Work out the finished part from the listing and answer in its coordinate system (mm). A direction names the side the tool comes from. Round coordinates to 2 decimals unless told otherwise and drop trailing zeros. Loops run counter-clockwise (first coordinate to the right, second up) from the corner with the lowest first, then second, coordinate; pieces in that order, holes last. Notation, with made-up numbers: (22, 84) - (47, 84) arc R8 cw to (47, 89) - close; hole circle Ø4 at (42.25, 51.5). An arc over 180 degrees is marked (long way). Return JSON: item names as keys, results as strings.
from build123d import *

# Parameters (mm, degrees)
BOSS_EXTRUDE1_DEPTH = 30
SKETCH2_R           = 1.5
SKETCH2_R_2         = 7.5
CUT_EXTRUDE1_DEPTH  = 14
SKETCH3_R           = 1.5
CUT_EXTRUDE2_DEPTH  = 76
FILLET1_R           = 5


with BuildPart() as part:
    # Sketch1 → Boss-Extrude1 (new body)
    with BuildSketch(Plane(origin=(0, 0, 0), x_dir=(1, 0, 0), z_dir=(0, 1, 0))):
        Polygon((-11.5, 4), (-1.5, 4), (-1.5, 75), (1.5, 75), (1.5, 4), (11.5, 4), (11.5, 0), (-11.5, 0), align=None)
    extrude(amount=BOSS_EXTRUDE1_DEPTH)

    # Sketch2 → Cut-Extrude1 (cut, through all)
    with BuildSketch(Plane.ZY.offset(1.5)):
        with Locations((-67.5, 15)):
            Circle(SKETCH2_R)
        with Locations((-31.5, 15)):
            Circle(SKETCH2_R)
        with Locations((-49.5, 15)):
            Circle(SKETCH2_R_2)
    extrude(amount=-CUT_EXTRUDE1_DEPTH, mode=Mode.SUBTRACT)

    # Sketch3 → Cut-Extrude2 (cut, through all)
    with BuildSketch(Plane.XY):
        with Locations((-6.5, 26)):
            Circle(SKETCH3_R)
        with Locations((-6.5, 4)):
            Circle(SKETCH3_R)
        with Locations((6.5, 4)):
            Circle(SKETCH3_R)
        with Locations((6.5, 26)):
            Circle(SKETCH3_R)
    extrude(amount=-CUT_EXTRUDE2_DEPTH, mode=Mode.SUBTRACT)

    # Fillet1
    fillet1_edges = [part.edges().sort_by_distance(p)[0] for p in [
        (11.5, 0, -2),
        (-11.5, 0, -2),
        (11.5, 30, -2),
        (0, 30, -75),
        (-11.5, 30, -2),
        (0, 0, -75),
    ]]
    fillet(fillet1_edges, radius=FILLET1_R)


solid = part.part
1) Section A-A (z = -67.5) is taken. Give the vertices of the cut face in (x, y), and give its area (3 significant figures).
Verdict:
{"outline": "(-1.5, 0) - (1.5, 0) - (1.5, 13.5) - (-1.5, 13.5) - close; (-1.5, 16.5) - (1.5, 16.5) - (1.5, 30) - (-1.5, 30) - close", "area": "81.0 mm2"}
2) Section B-B (y = 15) is taken. Give the vertices of the cut face in (x, z).
Verdict:
{"outline": "(-11.5, -4) - (-1.5, -4) - (-1.5, -30) - (1.5, -30) - (1.5, -4) - (11.5, -4) - (11.5, 0) - (-11.5, 0) - close; (-1.5, -75) - (1.5, -75) - (1.5, -69) - (-1.5, -69) - close; (-1.5, -66) - (1.5, -66) - (1.5, -57) - (-1.5, -57) - close; (-1.5, -42) - (1.5, -42) - (1.5, -33) - (-1.5, -33) - close"}
3) Flat-ended cylindrical pins translate along their axes: pin 1 (8 mm diameter, centred on y = 23, z = -66.5, fed in from +X); pin 2 (5 mm diameter, centred on x = 6.5, y = 26, fed in from -Z); pin 3 (3 mm diameter, centred on y = 20, z = -39.5, fed in from -X). Find the tip coordinate at first contact, or state that the pin passes through.
Verdict:
{"pin 1": "stops at x = 1.5", "pin 2": "stops at z = -4", "pin 3": "stops at x = -1.5"}
4) Section D-D (y = 4) is taken. Give the vertices of the cut face in (x, z).
Verdict:
{"outline": "(-11.4, -4) - (-8, -4) - (-8, 0) - (-11.4, 0) - close; (-5, -4) - (-1.5, -4) - (-1.5, -74.9) - (1.5, -74.9) - (1.5, -4) - (5, -4) - (5, 0) - (-5, 0) - close; (8, -4) - (11.4, -4) - (11.4, 0) - (8, 0) - close"}
5) Find the intervals of material crossed by L1, parallel to Y at x = 0.5, z = -67.5; L2, parallel to Y at x = -0.7, z = -49.5; L3, parallel to Z at x = 4.5, y = 6, in increasing order.
Verdict:
{"L1": "y = 0 to 13.5, 16.5 to 30", "L2": "y = 0 to 7.5, 22.5 to 30", "L3": "z = -4 to 0"}
6) Determine the mould class of faces 4 (the cylindrical face through (-6.695, 27.487, -1.972)), 5 (the flat face through (-1.5, 15, -39)), 6 (the flat face through (0, 30, -33)) for opening direction Y: pulls with the +Y half, pulls with the -Y half, needs draft (parallel to the pull), parting line crosses it, or undercut.
Verdict:
{"face 4": "undercut", "face 5": "needs draft", "face 6": "pulls with the +Y half"}
7) Section C-C (x = 0.25) is taken. Give the vertices of the cut face in (y, z).
Verdict:
{"outline": "(0, -70) arc R5 ccw to (5, -75) - (25, -75) arc R5 ccw to (30, -70) - (30, 0) - (0, 0) - close; hole circle Ø15 at (15, -49.5); hole circle Ø3 at (15, -67.5); hole circle Ø3 at (15, -31.5)"}
8) A tool of negligible diameter and unlimited length cuts with its end or side. For faces 1 (the flat face through (0, 15, 0)), 2 (the flat face through (6, 15, -4)), 3 (the flat face through (-7, 15, -4)), from which of +Z, -Z, +X, -X, +Y, -Y can it reach the whole face along a straight path? Write none if from no direction.
Verdict:
{"face 1": "+Z, +X, -X, +Y, -Y", "face 2": "-Z, +X, +Y, -Y", "face 3": "-Z, -X, +Y, -Y"}
